Build history of the part. All positions in model axes, mm. Face numbers are marked on the shaded views. A direction names the side the tool comes from. Give positions to 0.01 mm unless a question says otherwise; leave off trailing zeros. Write each loop counter-clockwise with the first axis right and the second up, starting at its lowest first coordinate (ties: lowest second). Pieces come first, ordered by that corner, then holes. Notation, with made-up numbers: M -9.75,39.5 L 27.25,39.5 A35 ccw 27.25,71.5 Z; hole C -31.5,34 d5. An arc over 180 degrees is marked long. Return JSON: item names as keys, results as strings. Group by question number.
Q1. Band-saw the part on B-B, the plane z = 4.5. Give the cut face in (x, y), then the cut area to 3 significant figures.
Q2. Pull direction Z, two halves, no side cores. Call the marked faces 1, 2, 3 and 4: +Z half, -Z half, draft (parallel to the pull), parting line (faces both ways), or undercut.
Q3. Band-saw the part on A-A, the plane x = -46. Give the cut face in (y, z).
Q4. Band-saw the part on D-D, the plane z = 36.5. Give the cut face in (x, y).
Q5. Tool access for the marked faces 5, 6 and 7: list every direction of +Z, -Z, +X, -X, +Y, -Y with a clear straight run to the whole face (end or side of a thin tool).
Q6. Band-saw the part on C-C, the plane z = 44.5. Give the cut face in (x, y).
Q7. Wall check: probe 1 along Z at (x, y) = (0, 25); probe 2 along X at (y, z) = (35, 36); probe 3 along X at (y, z) = (25.75, 36.5). Give the ranges that are in metal, low to high.
Q8. Flat gauge pins, fed straight in: pin 1 Ø15 at (x, y) = (6, 80) entering from +Z; pin 2 Ø1 at (y, z) = (24.5, 44.5) entering from +X; pin 3 Ø1.5 at (y, z) = (68, 14) entering from +X; pin 4 Ø5.5 at (x, y) = (51, 4.5) entering from -Z. Where does each tip first touch, or does it go through?
from build123d import *

# Parameters (mm, degrees)
EXTRUDE_1_DEPTH          = 54
EXTRUDE_2_DEPTH          = 50
EXTRUDE_3_DEPTH          = 23
EXTRUDE_4_DEPTH          = 25
CUT_EXTRUDE_1_REACH      = 91.672
CUT_EXTRUDE_1_END_RADIUS = 19
SKETCH_2_R               = 6.5
CUT_EXTRUDE_2_REACH      = 111.16


with BuildPart() as part:
    # 草图1 → 凸台-拉伸1 (new body)
    with BuildSketch(Plane.XY):
        with BuildLine():
            Line((54, 13), (25.922962794, 13))
            ThreePointArc((25.922962794, 13), (15.231546212, 24.677925359), (0, 29))
            Line((0, 29), (0, 19))
            ThreePointArc((0, 19), (13.435028843, 13.435028843), (19, 0))
            Line((19, 0), (54, 0))
            Line((54, 0), (54, 13))
        make_face()
        with BuildLine():
            ThreePointArc((0, 29), (-15.231546212, 24.677925359), (-25.922962794, 13))
            Line((-25.922962794, 13), (-54, 13))
            Line((-54, 13), (-54, 0))
            Line((-54, 0), (-19, 0))
            ThreePointArc((-19, 0), (-13.435028843, 13.435028843), (0, 19))
            Line((0, 19), (0, 29))
        make_face()
    extrude(amount=EXTRUDE_1_DEPTH)

    # 草图1<3> → 凸台-拉伸2 (add)
    with BuildSketch(Plane.XY):
        with BuildLine():
            Line((25.922962794, 13), (20.654024341, 44))
            Line((20.654024341, 44), (0, 44))
            Line((0, 44), (0, 29))
            ThreePointArc((0, 29), (15.231546212, 24.677925359), (25.922962794, 13))
        make_face()
        with BuildLine():
            Line((0, 44), (-20.654024341, 44))
            Line((-20.654024341, 44), (-25.922962794, 13))
            ThreePointArc((-25.922962794, 13), (-15.231546212, 24.677925359), (0, 29))
            Line((0, 29), (0, 44))
        make_face()
    extrude(amount=EXTRUDE_2_DEPTH)

    # 草图1<5> → 凸台-拉伸3 (add)
    with BuildSketch(Plane.XY):
        with BuildLine():
            ThreePointArc((0, 61), (-11.460837745, 66.322748418), (-14.78792136, 78.513440241))
            Line((-14.78792136, 78.513440241), (-20.654024341, 44))
            Line((-20.654024341, 44), (0, 44))
            Line((0, 44), (0, 61))
        make_face()
        with BuildLine():
            Line((20.654024341, 44), (14.78792136, 78.513440241))
            ThreePointArc((14.78792136, 78.513440241), (14.946886305, 77.26118587), (15, 76))
            ThreePointArc((15, 76), (10.606601718, 65.393398282), (0, 61))
            Line((0, 61), (0, 44))
            Line((0, 44), (20.654024341, 44))
        make_face()
    extrude(amount=EXTRUDE_3_DEPTH)

    # 草图1<6> → 凸台-拉伸4 (add)
    with BuildSketch(Plane.XY):
        with BuildLine():
            ThreePointArc((14.78792136, 78.513440241), (9.677251582, 87.460837745), (0, 91))
            Line((0, 91), (0, 84.5))
            ThreePointArc((0, 84.5), (6.01040764, 82.01040764), (8.5, 76))
            ThreePointArc((8.5, 76), (6.01040764, 69.98959236), (0, 67.5))
            Line((0, 67.5), (0, 61))
            ThreePointArc((0, 61), (10.606601718, 65.393398282), (15, 76))
            ThreePointArc((15, 76), (14.946886305, 77.26118587), (14.78792136, 78.513440241))
        make_face()
        with BuildLine():
            Line((0, 84.5), (0, 91))
            ThreePointArc((0, 91), (-9.677251582, 87.460837745), (-14.78792136, 78.513440241))
            ThreePointArc((-14.78792136, 78.513440241), (-11.460837745, 66.322748418), (0, 61))
            Line((0, 61), (0, 67.5))
            ThreePointArc((0, 67.5), (-8.5, 76), (0, 84.5))
        make_face()
    extrude(amount=EXTRUDE_4_DEPTH)

    # 切除-拉伸1: up to this cylinder (the profile starts outside it)
    cut_extrude_1_end = Plane(origin=(0, 0, 36.5), z_dir=(0, 0, -1)) * Cylinder(CUT_EXTRUDE_1_END_RADIUS, 222.344, mode=Mode.PRIVATE)
    # 草图2 → 切除-拉伸1 (cut, up to the surface)
    with BuildSketch(Plane(origin=(0, 44, 0), x_dir=(1, 0, 0), z_dir=(0, 1, 0)), mode=Mode.PRIVATE) as cut_extrude_1_sk1:
        with Locations(Location((0, -36.5, 0), (0, 0, 180))):
            Circle(SKETCH_2_R)
    cut_extrude_1_tool1 = extrude(cut_extrude_1_sk1.sketch, amount=-CUT_EXTRUDE_1_REACH, mode=Mode.PRIVATE) - cut_extrude_1_end
    add(cut_extrude_1_tool1.solids().sort_by_distance((0, 44, 36.5))[0], mode=Mode.SUBTRACT)

    # 草图3 → 切除-拉伸2 (cut, up to next)
    with BuildSketch(Plane(origin=(0, 13, 0), x_dir=(1, 0, 0), z_dir=(0, 1, 0)), mode=Mode.PRIVATE) as cut_extrude_2_sk1:
        with BuildLine():
            Line((-43, -22.5), (-54, -22.5))
            Line((-54, -22.5), (-54, -31.5))
            Line((-54, -31.5), (-43, -31.5))
            ThreePointArc((-43, -31.5), (-38.5, -27), (-43, -22.5))
        make_face()
    cut_extrude_2_tool1 = extrude(cut_extrude_2_sk1.sketch, amount=-CUT_EXTRUDE_2_REACH, mode=Mode.PRIVATE) & part.part
    # 草图3 → 切除-拉伸2 (cut, up to next)
    with BuildSketch(Plane(origin=(0, 13, 0), x_dir=(1, 0, 0), z_dir=(0, 1, 0)), mode=Mode.PRIVATE) as cut_extrude_2_sk2:
        with BuildLine():
            Line((54, -22.5), (54, -31.5))
            Line((54, -31.5), (43, -31.5))
            ThreePointArc((43, -31.5), (38.5, -27), (43, -22.5))
            Line((43, -22.5), (54, -22.5))
        make_face()
    cut_extrude_2_tool2 = extrude(cut_extrude_2_sk2.sketch, amount=-CUT_EXTRUDE_2_REACH, mode=Mode.PRIVATE) & part.part
    add(cut_extrude_2_tool1.solids().sort_by_distance((-46.698151, 13, 27))[0], mode=Mode.SUBTRACT)
    add(cut_extrude_2_tool2.solids().sort_by_distance((46.698151, 13, 27))[0], mode=Mode.SUBTRACT)


solid = part.part
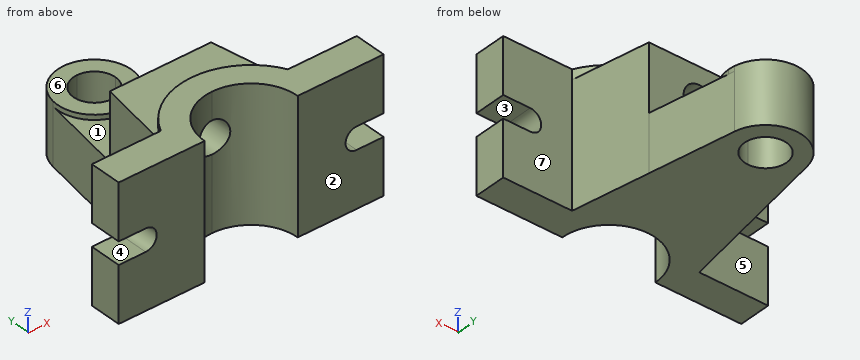
From the geometry:
{
 "1": {"outline": "M -54,0 L -19,0 A19 cw 19,0 L 54,0 L 54,13 L 25.92,13 L 14.79,78.51 A15 ccw -14.79,78.51 L -25.92,13 L -54,13 Z; hole C 0,76 d17", "area": "3,560 mm^2"},
 "2": {"face 1": "+Z half", "face 2": "draft", "face 3": "undercut", "face 4": "undercut"},
 "3": {"outline": "M 0,0 L 13,0 L 13,22.5 L 0,22.5 Z; M 0,31.5 L 13,31.5 L 13,54 L 0,54 Z"},
 "4": {"outline": "M -54,0 L -19,0 A19 cw -6.5,17.85 L -6.5,44 L -20.65,44 L -25.92,13 L -54,13 Z; M 6.5,17.85 A19 cw 19,0 L 54,0 L 54,13 L 25.92,13 L 20.65,44 L 6.5,44 Z"},
 "5": {"face 5": "+Z, -Z, -X, +Y", "face 6": "+Z, +X, -X, +Y", "face 7": "+Z, -Z, +X, +Y"},
 "6": {"outline": "M -54,0 L -19,0 A19 cw 19,0 L 54,0 L 54,13 L 25.92,13 L 20.65,44 L -20.65,44 L -25.92,13 L -54,13 Z"},
 "7": {"probe 1": "z = 0 to 30, 43 to 54", "probe 2": "x = -22.18 to -6.48, 6.48 to 22.18", "probe 3": "x = -23.76 to -6.5, 6.5 to 23.76"},
 "8": {"pin 1": "stops at z = 25", "pin 2": "stops at x = 24.05", "pin 3": "stops at x = 16.7", "pin 4": "stops at z = 0"}
}
